Work out the finished part from the listing and answer in its coordinate system (mm). Face numbers are marked on the shaded views. A direction names the side the tool comes from. Round coordinates to 2 decimals unless told otherwise and drop trailing zeros. Order: outer loops, then holes, each group sorted by start corner. A loop starts at its lowest first (then second) coordinate and runs counter-clockwise, first axis right, second up. Notation, with made-up numbers: M -27,42.5 L -4,42.5 A10 cw -4,57.5 Z; hole C 21,-21.5 d8. An arc over 180 degrees is marked long. Answer as a JSON object with one key per item and string values. Group by question number.
Autodesk Inventor part; units mm, degrees
ref_plane "Work Plane1" through (-165, 90, 5) normal (0, 1, 0) x (1, 0, 0)
ref_plane "YZ Plane" through (0, 0, 0) normal (1, 0, 0) x (0, 1, 0)
ref_plane "XZ Plane" through (0, 0, 0) normal (0, 1, 0) x (-1, 0, 0)
sketch "Sketch1" plane through (0, 0, 0) normal (0, 0, 1) x (1, 0, 0)
  line L0 (0, 0) -> (-44, 0)
  line L1 (-44, 0) -> (-44, 90)
  line L2 (-44, 90) -> (0, 90)
  line L3 (0, 90) -> (0, 0)
  line L4 (-44, 90) -> (-165, 90)
  line L5 (-165, 90) -> (-165, 50)
  line L6 (-165, 50) -> (-44, 50)
  line L7 (-44, 50) -> (-44, 90)
  point P0 (-44, 50)
  dimension "d0" = 44
  dimension "d1" = 90
  dimension "d2" = 40
  dimension "d3" = 121
extrude "Extrusion1" add sketch "Sketch1" along normal blind 5
sketch "Sketch2" plane through (0, 0, 5) normal (0, 0, 1) x (1, 0, 0)
  point P0 (0, 0)
ref_plane "Work Plane1" through (-165, 90, 5) normal (0, 1, 0) x (1, 0, 0)
sketch "Sketch3" plane through (-165, 90, 5) normal (0, 1, 0) x (1, 0, 0)
  circle A0 centre (150, -25) radius 15
  arc A1 (7.1929, -25.7193) -> (7.1925, -24.2771) centre (0, -25) ccw
  line L0 (165, 0) -> (0.2186, 0)
  line L1 (165, 5) -> (165, -44.7143)
  line L2 (150, -40) -> (0, -25)
  line L3 (0, -25) -> (148.5, -10.0752)
  line L4 (0, 0) -> (121, 0)
  line L5 (165, -44.7143) -> (0, -44.7143)
  line L6 (0, -44.7143) -> (0, 0)
  line L7 (0, 0) -> (165, 0)
  line L8 (165, 0) -> (165, -44.7143)
  line L9 (0, 0) -> (0, -44.7143)
  point P0 (0, -25)
  point P1 (165, -25)
  dimension "d6" = 30
  dimension "d7" = 150
  dimension "d8" = 165
  dimension "d9" = 25
extrude "Extrusion2" add sketch "Sketch3" against normal blind 10 contours A0 L3 L6 L4 L0 L1
sketch "Sketch4" plane through (0, 0, 5) normal (0, 0, 1) x (1, 0, 0)
  line L0 (-5, 5) -> (-15, 5)
  line L1 (-15, 5) -> (-15, 15)
  line L2 (-15, 15) -> (-5, 15)
  line L3 (-5, 15) -> (-5, 5)
  line L4 (-5, 5) -> (-15, 15) construction
  line L5 (-15, 5) -> (-5, 15) construction
  line L6 (-44, 0) -> (0, 0)
  line L7 (0, 0) -> (0, 80)
  line L8 (-22, 0) -> (-22, 96.74)
  line L9 (0, 80) -> (-165, 80)
  line L10 (-39, 5) -> (-29, 5)
  line L11 (-29, 5) -> (-29, 15)
  line L12 (-29, 15) -> (-39, 15)
  line L13 (-39, 15) -> (-39, 5)
  line L14 (-5, 65) -> (-15, 65)
  line L15 (-15, 65) -> (-15, 75)
  line L16 (-15, 75) -> (-5, 75)
  line L17 (-5, 75) -> (-5, 65)
  line L18 (-5, 65) -> (-15, 75) construction
  line L19 (-15, 65) -> (-5, 75) construction
  line L20 (-39, 65) -> (-29, 65)
  line L21 (-29, 65) -> (-29, 75)
  line L22 (-29, 75) -> (-39, 75)
  line L23 (-39, 75) -> (-39, 65)
  line L24 (-140, 60) -> (-150, 60)
  line L25 (-150, 60) -> (-150, 70)
  line L26 (-150, 70) -> (-140, 70)
  line L27 (-140, 70) -> (-140, 60)
  line L28 (-140, 60) -> (-150, 70) construction
  line L29 (-150, 60) -> (-140, 70) construction
  line L30 (-165, 50) -> (-44, 50)
  line L31 (-165, 80) -> (-165, 50)
  circle A0 centre (-10, 10) radius 1.5
  circle A1 centre (-10, 70) radius 1.5
  circle A2 centre (-34, 10) radius 1.5
  circle A3 centre (-34, 70) radius 1.5
  circle A4 centre (-145, 65) radius 1.5
  dimension "d12" = 10
  dimension "d13" = 10
  dimension "d14" = 10
  dimension "d15" = 10
  dimension "d16" = 10
  dimension "d17" = 10
  dimension "d18" = 10
  dimension "d19" = 10
  dimension "d20" = 10
  dimension "d21" = 15
  dimension "d22" = 20
  dimension "d23" = 3
  dimension "d24" = 3
  dimension "d25" = 3
extrude "Extrusion3" cut sketch "Sketch4" against normal through all contours A0 | A1
extrude "Extrusion4" cut sketch "Sketch4" against normal through all contours A3
extrude "Extrusion5" cut sketch "Sketch4" against normal through all contours A2
extrude "Extrusion6" cut sketch "Sketch4" against normal through all contours A4
sketch "Sketch5" plane through (0, 0, 0) normal (0, 0, -1) x (-1, 0, 0)
  line L0 (5, 15) -> (15, 15)
  line L1 (15, 15) -> (15, 5)
  line L2 (15, 5) -> (5, 5)
  line L3 (5, 5) -> (5, 15)
  circle A0 centre (10, 10) radius 1.5
  line L4 (5, 15) -> (15, 5) construction
  line L5 (15, 15) -> (5, 5) construction
  line L6 (5, 75) -> (15, 75)
  line L7 (15, 75) -> (15, 65)
  line L8 (15, 65) -> (5, 65)
  line L9 (5, 65) -> (5, 75)
  circle A1 centre (10, 70) radius 1.5
  line L10 (5, 75) -> (15, 65) construction
  line L11 (15, 75) -> (5, 65) construction
  line L12 (44, 0) -> (0, 0)
  line L13 (22, 0) -> (22, 89.9769)
  line L14 (39, 15) -> (29, 15)
  line L15 (29, 15) -> (29, 5)
  line L16 (29, 5) -> (39, 5)
  line L17 (39, 5) -> (39, 15)
  circle A2 centre (34, 10) radius 1.5
  line L18 (39, 15) -> (29, 5) construction
  line L19 (29, 15) -> (39, 5) construction
  line L20 (39, 75) -> (29, 75)
  line L21 (29, 75) -> (29, 65)
  line L22 (29, 65) -> (39, 65)
  line L23 (39, 65) -> (39, 75)
  circle A3 centre (34, 70) radius 1.5
  line L24 (39, 75) -> (29, 65) construction
  line L25 (29, 75) -> (39, 65) construction
  line L26 (140, 70) -> (150, 70)
  line L27 (150, 70) -> (150, 60)
  line L28 (150, 60) -> (140, 60)
  line L29 (140, 60) -> (140, 70)
  circle A4 centre (145, 65) radius 1.5
  line L30 (140, 70) -> (150, 60) construction
  line L31 (150, 70) -> (140, 60) construction
  circle A5 centre (10, 10) radius 1.5
  circle A6 centre (10, 70) radius 1.5
  circle A7 centre (34, 70) radius 1.5
  circle A8 centre (34, 10) radius 1.5
  circle A9 centre (145, 65) radius 1.5
  dimension "d34" = 10
  dimension "d35" = 10
  dimension "d36" = 10
  dimension "d37" = 10
  dimension "d38" = 10
  dimension "d39" = 10
  dimension "d40" = 3
  dimension "d41" = 3
  dimension "d42" = 3
  dimension "d43" = 3
  dimension "d44" = 3
extrude "Extrusion7" cut sketch "Sketch5" against normal blind 2
properties part number "üst kısım"
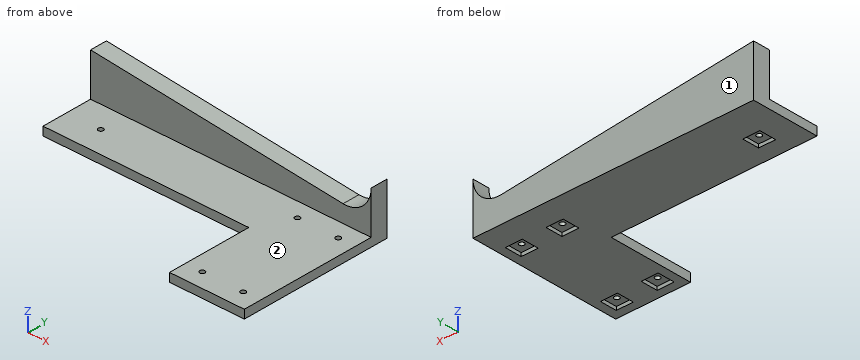
Item 1: Each of these flat-tipped pins is pushed along its axis until it touches: pin 1 (2 mm diameter, centred on y = 9.5, z = 1, fed in from -X); pin 2 (1.5 mm diameter, centred on x = -138.5, y = 55, fed in from +Z); pin 3 (3 mm diameter, centred on x = -145.5, y = 65.5, fed in from -Z). Where does it stop, or does it pass through?
Item 2: A tool of negligible diameter and unlimited length cuts with its end or side. For the marked faces 1 and 2, from which of +Z, -Z, +X, -X, +Y, -Y can it reach the whole face along a straight path? Write none if from no direction.
Item 3: Find section A-A (z = 23.5). Give the vertices of the cut face in (x, y), and give its area (3 significant figures).
Item 4: Consider L1, parallel to X at y = 10, z = 3.7; L2, parallel to Y at x = -34, z = 2.65; L3, parallel to X at y = 70, z = 4. Determine where each line is inside the solid, lowest interval first.
Item 5: Find section B-B (y = 28). Give the vertices of the cut face in (x, z), and give its area (3 significant figures).
Responses:
{
 "1": {"pin 1": "stops at x = -44", "pin 2": "stops at z = 5", "pin 3": "stops at z = 2"},
 "2": {"face 1": "+Z, -Z, +X, -X, +Y", "face 2": "+Z, +X, -X, -Y"},
 "3": {"outline": "M -165,80 L -100.33,80 L -100.33,90 L -165,90 Z; M -1.48,80 L 0,80 L 0,90 L -1.48,90 Z", "area": "662 mm^2"},
 "4": {"L1": "x = -44 to -35.5, -32.5 to -11.5, -8.5 to 0", "L2": "y = 0 to 8.5, 11.5 to 68.5, 71.5 to 90", "L3": "x = -165 to -35.5, -32.5 to -11.5, -8.5 to 0"},
 "5": {"outline": "M -44,0 L 0,0 L 0,5 L -44,5 Z", "area": "220 mm^2"}
}
